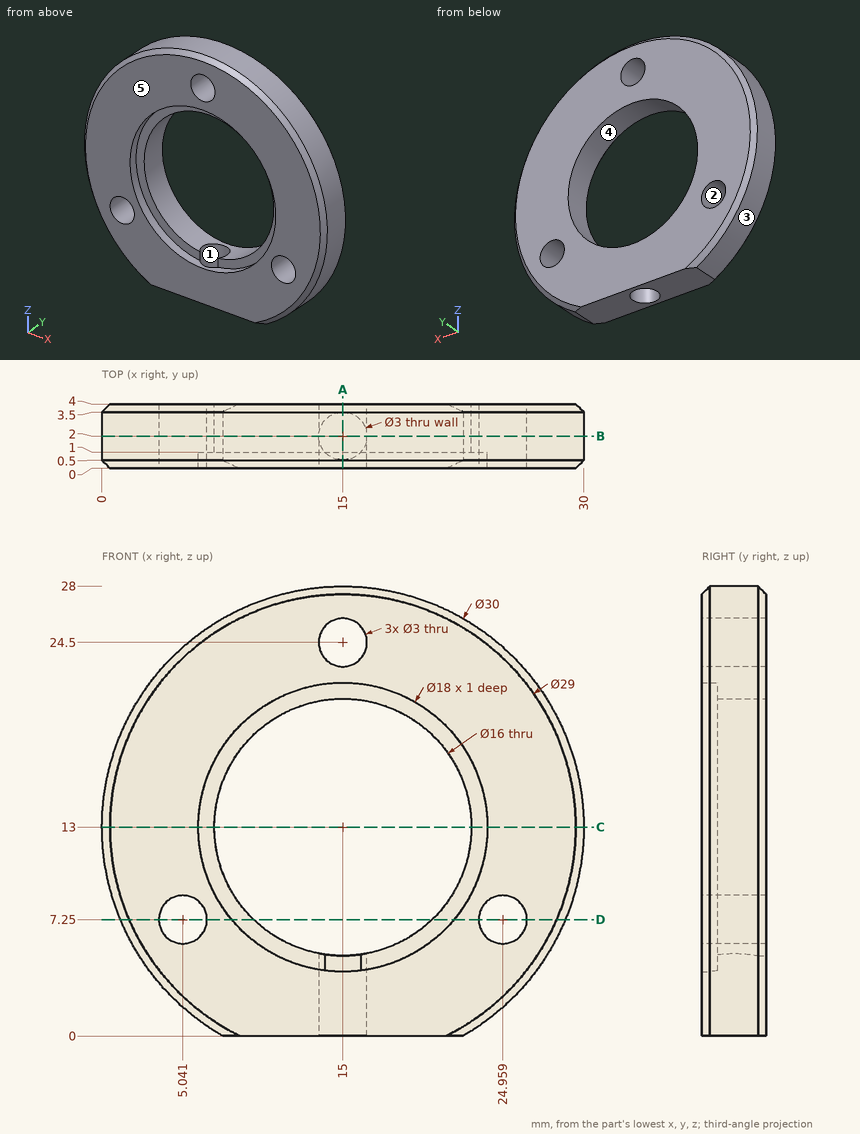
Source: three-view drawing plus pictorial views. Frame: mm from the lowest corner of the part. A direction names the side the tool comes from. Give positions to 0.01 mm unless a question says otherwise; leave off trailing zeros. Write each loop counter-clockwise with the first axis right and the second up, starting at its lowest first coordinate (ties: lowest second). Pieces come first, ordered by that corner, then holes. Notation, with made-up numbers: (16, -5.75) - (72, -5.75) arc R22 cw to (72, 11.25) - close; hole circle Ø4 at (-6, -13.75). An arc over 180 degrees is marked (long way). Write item = value, one per line. Start each with the question number.
1. Section query A-A, the plane x = 15. Output: boundary loops of the cut face in (y, z).
2. Mould query, pull axis X, two halves, no side actions, for the marked faces 3, 4 and 5. Classes: released by +X, released by -X, zero draft, split by the parting line, or undercut.
3. First-contact query: pin 1 Ø2.5 at (x, z) = (24.96, 7.25) entering from -Y; pin 2 Ø1.5 at (y, z) = (1.5, 24.5) entering from +X; pin 3 Ø9 at (x, z) = (18, 10) entering from -Y; pin 4 Ø5 at (x, z) = (8.5, 15.5) entering from +Y. Flat tips, straight axial feed; report the tip coordinate or a pass-through.
4. Section query C-C, the plane z = 13. Output: boundary loops of the cut face in (x, y).
5. Section query D-D, the plane z = 7.25. Count the separate pieces of the cut face and the enclosed holes in it.
6. Access query for the marked faces 1 and 2. Directions: +Z, -Z, +X, -X, +Y, -Y. A direction counts if a zero-diameter tool reaches every point of the face in a straight line with its end or side. Return the directions, or none.
7. Ray query, L1, parallel to Z at x = 15, y = 1.7; L2, parallel to Y at x = 15, z = 4.05; L3, parallel to Z at x = 26.25, y = 0.9 (1 decimal). Return the intervals inside material, ascending.
8. Section query B-B, the plane y = 2. Output: boundary loops of the cut face in (x, z), then the cut area to 3 significant figures.
Check sheet entries:
q1.outline = (0, 0) - (0.5, 0) - (0.5, 4) - (0, 4) - close; (0, 22) - (1, 22) - (1, 21) - (4, 21) - (4, 23) - (0, 23) - close; (0, 26) - (4, 26) - (4, 27.5) - (3.5, 28) - (0.5, 28) - (0, 27.5) - close; (3.5, 0) - (4, 0) - (4, 5) - (3.5, 5) - close
q2.face_3 = split by the parting line
q2.face_4 = undercut
q2.face_5 = zero draft
q3.pin_1 = through
q3.pin_2 = 25.46
q3.pin_3 = 1
q3.pin_4 = 4
q4.outline = (0, 0.5) - (0.5, 0) - (6, 0) - (6, 1) - (7, 1) - (7, 4) - (0.5, 4) - (0, 3.5) - close; (23, 1) - (24, 1) - (24, 0) - (29.5, 0) - (30, 0.5) - (30, 3.5) - (29.5, 4) - (23, 4) - close
q5.separate_pieces = 4
q5.enclosed_holes = 0
q6.face_1 = -Z
q6.face_2 = +Y, -Y
q7.L1 = 21 to 23, 26 to 28
q7.L2 = 3.5 to 4
q7.L3 = 3.1 to 6.5, 8 to 22.9
q8.outline = (7.52, 0) - (13.5, 0) - (13.5, 5.14) arc R8 cw (long way) to (16.5, 5.14) - (16.5, 0) - (22.48, 0) arc R15 ccw (long way) to start; hole circle Ø3 at (5.04, 7.25); hole circle Ø3 at (15, 24.5); hole circle Ø3 at (24.96, 7.25)
q8.area = 449 mm2
